Geometry check sheet. Reference: drawing and pictorial views, mm from the part's lowest x, y, z. Give positions to 0.01 mm unless a question says otherwise; leave off trailing zeros. Order: outer loops, then holes, each group sorted by start corner. A loop starts at its lowest first (then second) coordinate and runs counter-clockwise, first axis right, second up. Notation, with made-up numbers: M 82,30 L 141,30 A18 ccw 141,40 Z; hole C -7,-26 d7. An arc over 180 degrees is marked long. Answer as CSV lines item,"result".
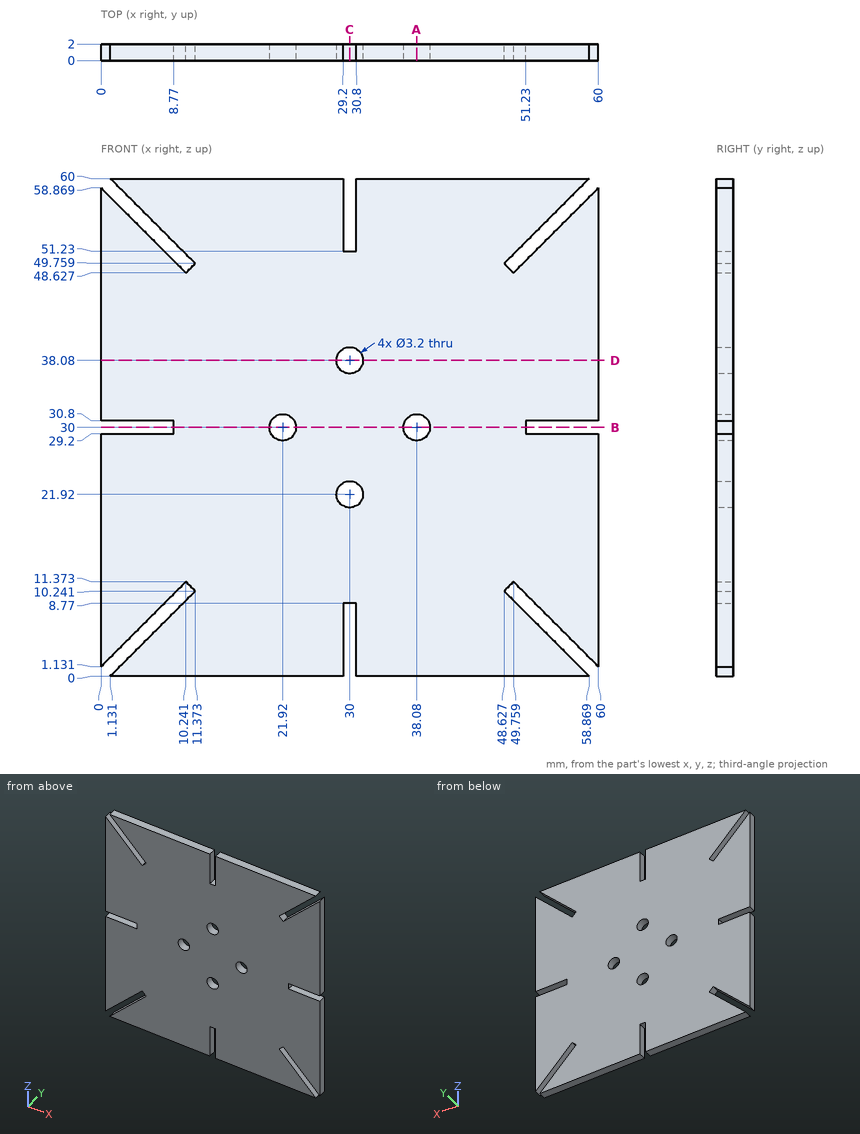
(1) Material ranges on line 1 (X direction, y = 0.6, z = 30); line 2 (X direction, y = 0.25, z = 52); line 3 (X direction, y = 0.45, z = 38.08), recorded low to high.
The answers:
line 1,"x = 8.77 to 20.32, 23.52 to 36.48, 39.68 to 51.23"
line 2,"x = 0 to 6.87, 9.13 to 29.2, 30.8 to 50.87, 53.13 to 60"
line 3,"x = 0 to 28.4, 31.6 to 60"
(2) Section check B-B on z = 30. Enter the section's corners in (x, y).
The answers:
outline,"M 8.77,0 L 20.32,0 L 20.32,2 L 8.77,2 Z; M 23.52,0 L 36.48,0 L 36.48,2 L 23.52,2 Z; M 39.68,0 L 51.23,0 L 51.23,2 L 39.68,2 Z"
(3) Section check A-A on x = 38.08. Enter the section's corners in (y, z).
The answers:
outline,"M 0,0 L 2,0 L 2,28.4 L 0,28.4 Z; M 0,31.6 L 2,31.6 L 2,60 L 0,60 Z"
(4) Section check C-C on x = 30. Enter the section's corners in (y, z).
The answers:
outline,"M 0,8.77 L 2,8.77 L 2,20.32 L 0,20.32 Z; M 0,23.52 L 2,23.52 L 2,36.48 L 0,36.48 Z; M 0,39.68 L 2,39.68 L 2,51.23 L 0,51.23 Z"
(5) Gauge pin test, flat end, axial feed: P1, Ø1.9, axis at x = 21.92, z = 30, coming from the -Y side. Record the tip position at first contact, or that the pin passes through.
The answers:
P1,"passes through"
(6) Section check D-D on z = 38.08. Enter the section's corners in (x, y).
The answers:
outline,"M 0,0 L 28.4,0 L 28.4,2 L 0,2 Z; M 31.6,0 L 60,0 L 60,2 L 31.6,2 Z"
